Verification items for the finished model (mm, model axes). Coordinates: 2 decimals unless noted, no trailing zeros. Order: outer loops, then holes, each group sorted by start corner. A loop starts at its lowest first (then second) coordinate and runs counter-clockwise, first axis right, second up. Notation, with made-up numbers: M 43.25,-35 L 65.25,-35 A27 ccw 65.25,-13 Z; hole C 21,-13 d4. An arc over 180 degrees is marked long. Answer as a JSON object with one key per item and string values. Group by question number.
(1) Gauge pin test, flat ends, axial feed: pin 1 Ø2.5 at (x, y) = (-171.24, -34.32) entering from -Z; pin 2 Ø2 at (y, z) = (-105, 2.5) entering from +X; pin 3 Ø3 at (y, z) = (-104.5, 1.5) entering from -X. Record the tip position at first contact, or that the pin passes through.
(2) Material ranges on line 1 (X direction, y = -4, z = 2.75); line 2 (X direction, y = -25.5, z = 1); line 3 (Y direction, x = -172, z = 2.25), recorded low to high.
(3) Cross-section at A-A (y = -11.5). Enter the section's corners in (x, z), plus the area to 3 significant figures.
(4) Cross-section at B-B (x = -219). Enter the section's corners in (y, z).
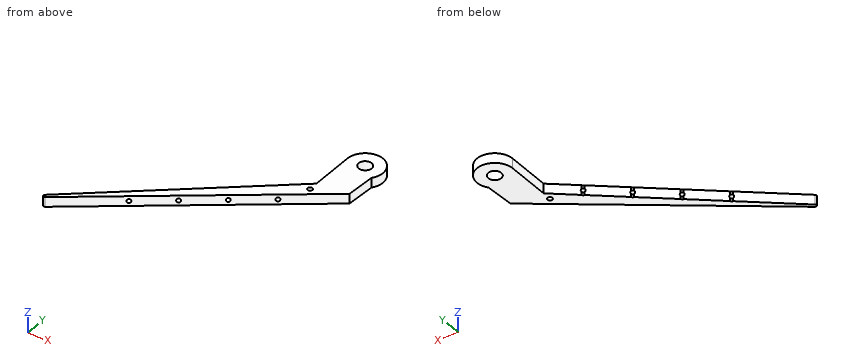
Autodesk Inventor part; units mm, degrees
ref_plane "YZ Plane" through (0, 0, 0) normal (1, 0, 0) x (0, 1, 0)
ref_plane "XZ Plane" through (0, 0, 0) normal (0, 1, 0) x (-1, 0, 0)
ref_plane "XY Plane" through (0, 0, 0) normal (0, 0, 1) x (1, 0, 0)
sketch "スケッチ1" plane through (0, 0, 0) normal (0, 0, 1) x (1, 0, 0)
  circle A0 centre (-149.101, -13.3308) radius 1.5 construction
  circle A1 centre (-160.5892, -1.6149) radius 1.5 construction
  circle A2 centre (-44.4492, 64.0137) radius 1.5 construction
  circle A3 centre (-64.4423, 49.0046) radius 1.5 construction
  circle A4 centre (-60.4494, 64.5064) radius 1.5 construction
  arc A5 (-40.2316, 58.3956) -> (-44.233, 71.0354) centre (-44.4492, 64.0137) ccw construction
  line L0 (-44.233, 71.0354) -> (-60.2332, 71.5281) construction
  arc A6 (-60.2332, 71.5281) -> (-64.1725, 70.4637) centre (-60.4494, 64.5064) ccw construction
  line L1 (-64.1725, 70.4637) -> (-165.9022, 6.8864) construction
  arc A7 (-165.9022, 6.8864) -> (-166.8262, -9.4635) centre (-160.5892, -1.6149) ccw construction
  line L2 (-166.8262, -9.4635) -> (-154.0782, -19.594) construction
  arc A8 (-154.0782, -19.594) -> (-144.2981, -19.7286) centre (-149.101, -13.3308) ccw construction
  line L3 (-144.2981, -19.7286) -> (-40.2316, 58.3956) construction
  circle A9 centre (-82.1645, 51.5544) radius 1.5 construction
  circle A10 centre (-141.748, 14.817) radius 1.5 construction
  circle A11 centre (-89.4637, 29.5642) radius 1.5 construction
  circle A12 centre (-117.4541, 8.5514) radius 1.5 construction
  circle A13 centre (-111.8449, 33.0052) radius 1.5 construction
  line L4 (-152.7009, -26.0367) -> (-305.9655, -141.0946)
  circle A14 centre (-149.101, -13.3308) radius 1.5 construction
  circle A15 centre (-149.101, -13.3308) radius 3 construction
  circle A16 centre (-149.101, -13.3308) radius 3 construction
  circle A17 centre (-160.5892, -1.6149) radius 9.025 construction
  circle A18 centre (-160.5892, -1.6149) radius 4.025
  line L5 (-152.7009, -26.0367) -> (-151.5741, -2.0382)
  line L6 (-64.1725, 70.4637) -> (-165.9022, 6.8864) construction
  line L7 (-144.2981, -19.7286) -> (-40.2316, 58.3956) construction
  line L8 (-305.9655, -141.0946) -> (-171.4423, -28.6314)
  line L9 (-160.5892, -1.6149) -> (-146.0204, -21.0215) construction
  line L10 (-146.0204, -21.0215) -> (-305.9655, -141.0946) construction
  circle A19 centre (-276.0256, -117.3678) radius 1
  circle A20 centre (-160.5892, -1.6149) radius 11
  line L11 (-171.4423, -28.6314) -> (-171.589, -1.6748)
  point P0 (0, 0)
  point P1 (0, 0)
  point P2 (-276.667, -116.6006)
  point P3 (-275.4252, -118.1676)
  point P4 (-151.8691, -8.3201)
  dimension "d6" = 22
  dimension "d0" = 6
  dimension "d1" = 8.05
  dimension "d2" = 5
  dimension "d3" = 3
  dimension "d4" = 200
  dimension "d5" = 2
  dimension "d7" = 3
  dimension "d8" = 6
extrude "押し出し1" add sketch "スケッチ1" along normal blind 6 contours L4 A19 L8 L11 A20 L5 | A19 | A20
sketch "スケッチ2" plane through (0, 0, 6) normal (0, 0, 1) x (1, 0, 0)
  line L0 (-171.589, -1.6748) -> (-171.4423, -28.6314)
  line L1 (-171.4423, -28.6314) -> (-276.667, -116.6006)
  arc A0 (-276.667, -116.6006) -> (-275.4252, -118.1676) centre (-276.0256, -117.3678) ccw
  line L2 (-275.4252, -118.1676) -> (-152.7009, -26.0367)
  line L3 (-152.7009, -26.0367) -> (-151.8691, -8.3201)
  arc A1 (-151.8691, -8.3201) -> (-171.589, -1.6748) centre (-160.5892, -1.6149) ccw
  circle A2 centre (-160.5892, -1.6149) radius 4.025
  circle A3 centre (-171.2358, -34.3242) radius 1.5
  circle A4 centre (-171.2358, -34.3242) radius 3
  circle A5 centre (-171.2358, -34.3242) radius 4.5
  point P0 (0, 0)
  dimension "d11" = 3
  dimension "d12" = 6
  dimension "d13" = 9
extrude "押し出し2" cut sketch "スケッチ2" against normal through all contours A3
sketch "スケッチ3" plane through (0, 0, 6) normal (0, 0, 1) x (1, 0, 0)
  line L0 (-171.4423, -28.6314) -> (-276.667, -116.6006)
  circle A0 centre (-244.7975, -88.9797) radius 1.05
  circle A1 centre (-225.6172, -72.9448) radius 1.05
  circle A2 centre (-206.437, -56.9099) radius 1.05
  circle A3 centre (-187.2568, -40.8749) radius 1.05
  point P0 (0, 0)
  dimension "d16" = 2.1
  dimension "d17" = 2.1
  dimension "d18" = 2.1
  dimension "d19" = 2.1
  dimension "d20" = 0.75
  dimension "d21" = 0.75
  dimension "d22" = 0.75
  dimension "d23" = 0.75
  dimension "d24" = 20
  dimension "d25" = 25
  dimension "d26" = 25
  dimension "d27" = 25
extrude "押し出し3" cut sketch "スケッチ3" against normal through all
sketch "スケッチ4" plane through (-205.3922, -57.0139, 6) normal (-0.6413971, 0.7672091, 0) x (0.7672091, 0.6413971, 0)
  line L0 (-25, 6) -> (-25, 0)
  line L1 (-1.4697, 0) -> (-25, 0)
  line L2 (-1.4697, 0) -> (-1.4697, 6)
  line L3 (-1.4697, 6) -> (-25, 6)
  line L4 (-26.4697, 0) -> (-26.4697, 6)
  line L5 (-26.4697, 6) -> (-50, 6)
  line L6 (-50, 6) -> (-50, 0)
  line L7 (-26.4697, 0) -> (-50, 0)
  line L8 (-51.4697, 0) -> (-51.4697, 6)
  line L9 (-51.4697, 6) -> (-92.9014, 6)
  line L10 (-92.9014, 6) -> (-92.9014, 0)
  line L11 (-51.4697, 0) -> (-92.9014, 0)
  line L12 (0, 6) -> (0, 0)
  line L13 (23.5303, 0) -> (0, 0)
  line L14 (23.5303, 0) -> (23.5303, 6)
  line L15 (23.5303, 6) -> (0, 6)
  line L16 (25, 6) -> (25, 0)
  line L17 (44.2511, 0) -> (25, 0)
  line L18 (44.2511, 6) -> (44.2511, 0)
  line L19 (44.2511, 6) -> (25, 6)
  circle A0 centre (-50.7348, 3) radius 1.25
  circle A1 centre (-25.7348, 3) radius 1.25
  circle A2 centre (-0.7348, 3) radius 1.25
  circle A3 centre (24.2652, 3) radius 1.25
  line L20 (23.5303, 6) -> (25, 6)
  line L21 (-1.4697, 6) -> (0, 6)
  line L22 (-26.4697, 6) -> (-25, 6)
  line L23 (-51.4697, 6) -> (-50, 6)
  point P0 (194.1473, 6)
  point P1 (-51.4697, 3)
  point P2 (-26.4697, 3)
  point P3 (-50.7348, 6)
  point P4 (-25.7348, 6)
  point P5 (-0.7348, 6)
  point P6 (24.2652, 6)
  point P7 (23.5303, 3)
  point P8 (-1.4697, 3)
  dimension "d30" = 2.5
  dimension "d31" = 2.5
  dimension "d32" = 2.5
  dimension "d33" = 2.5
extrude "押し出し4" cut sketch "スケッチ4" against normal through all contours A1 L0 | L0 A1 L4 | L4 A1 | A2 L12 L2 | L2 A2 | A2 L12 | A0 L6 | L6 A0 L8 | A3 L16 L14 | L14 A3 | L8 A0 | A3 L16
sketch "スケッチ5" plane through (0, 0, 6) normal (0, 0, 1) x (1, 0, 0)
  arc A0 (-225.7, -73.9915) -> (-224.5724, -73.0489) centre (-225.6172, -72.9448) ccw
  line L0 (-225.7, -73.9915) -> (-243.7526, -89.0838)
  arc A1 (-244.8802, -90.0264) -> (-243.7526, -89.0838) centre (-244.7975, -88.9797) ccw
  line L1 (-244.8802, -90.0264) -> (-276.667, -116.6006)
  arc A2 (-276.667, -116.6006) -> (-275.4252, -118.1676) centre (-276.0256, -117.3678) ccw
  line L2 (-275.4252, -118.1676) -> (-152.7009, -26.0367)
  line L3 (-152.7009, -26.0367) -> (-151.8691, -8.3201)
  arc A3 (-151.8691, -8.3201) -> (-171.589, -1.6748) centre (-160.5892, -1.6149) ccw
  line L4 (-171.589, -1.6748) -> (-171.4423, -28.6314)
  line L5 (-171.4423, -28.6314) -> (-186.2119, -40.979)
  arc A4 (-187.3395, -41.9217) -> (-186.2119, -40.979) centre (-187.2568, -40.8749) ccw
  line L6 (-187.3395, -41.9217) -> (-205.3922, -57.0139)
  arc A5 (-206.5197, -57.9566) -> (-205.3922, -57.0139) centre (-206.437, -56.9099) ccw
  line L7 (-206.5197, -57.9566) -> (-224.5724, -73.0489)
  circle A6 centre (-171.2358, -34.3242) radius 1.5
  circle A7 centre (-160.5892, -1.6149) radius 4.025
  point P0 (0, 0)
equation "\"d8\" = d0"
equation "\"d21\" = d20"
equation "\"d22\" = d21"
equation "\"d23\" = d21"
equation "\"d26\" = d25"
equation "\"d27\" = d26"
properties part number "アームシールド根本1" material "アルミニウム 7075"
Taken from the geometry:
{
 "1": {"pin 1": "passes through", "pin 2": "stops at x = -256.55", "pin 3": "stops at x = -263.99"},
 "2": {"line 1": "x = -171.58 to -163.83, -157.35 to -149.85", "line 2": "x = -171.46 to -152.68", "line 3": "y = -40.52 to -35.61, -33.03 to -29.1"},
 "3": {"outline": "M -171.54,0 L -152.02,0 L -152.02,6 L -171.54,6 Z", "area": "117 mm²"},
 "4": {"outline": "M -75.81,0 L -68.39,0 L -68.39,6 L -75.81,6 Z"}
}
